Geometry check sheet. Reference: the model listing, model coordinates, mm. A direction names the side the tool comes from. Coordinates: 2 decimals unless noted, no trailing zeros. Loops run counter-clockwise (first coordinate to the right, second up) from the corner with the lowest first, then second, coordinate; pieces in that order, holes last. Notation, with made-up numbers: (-22.75, 19) - (21.25, 19) arc R20 cw to (21.25, 56) - close; hole circle Ø7 at (-4.75, 72). An arc over 180 degrees is marked (long way). Write each question's results on one line, items separated by ' | '. Start each with the question number.
(1) Mould release check, pull along Y, two halves, no side actions. Record for faces 3 (the face through (31, 9.76, 11.83)), 4 (the face through (-25, 0, 23)), 5 (the face through (-29, -9, -3)): pulls with the +Y half, pulls with the -Y half, needs draft (parallel to the pull), parting line crosses it, or undercut.
(2) Sectioned sample at C-C (z = 8.75). Enter the section's corners in (x, y), plus the area to 3 significant figures.
(3) Access from +Z, -Z, +X, -X, +Y, -Y to the whole of each face (thin tool, end or side, straight path). Record for faces 1 (the face through (-28, 0, 21.5)), 2 (the face through (25, 0, 23)).
(4) Sectioned sample at D-D (y = 23). Enter the section's corners in (x, z).
(5) Material ranges on probe 1 along Y at (x, z) = (0, 11.5); probe 2 along Y at (x, z) = (27.5, 14.5); probe 3 along Z at (x, y) = (23.5, 24.5), recorded low to high.
(6) Go/stop test with flat-tipped pins: pin 1 Ø2.5 at (x, y) = (28.5, -1) entering from -Z; pin 2 Ø2 at (x, z) = (26.5, 22.5) entering from +Y; pin 3 Ø0.8 at (x, z) = (0, 23) entering from +Y. Record where each tip stops, or that it passes through.
(7) Sectioned sample at A-A (y = 0). Enter the section's corners in (x, z).
from build123d import *

# Parameters (mm, degrees)
F0_R     = 42.5
F0_R_2   = 32.5
F0_R_3   = 30
F1_DEPTH = 3
F2_DEPTH = 24
F4_DEPTH = 2.5


with BuildPart() as f1:
    # F0 (on Top) → F1 (new body)
    with BuildSketch(Plane.XY):
        Circle(F0_R)
        Circle(F0_R_2, mode=Mode.SUBTRACT)
        Circle(F0_R_2)
        Circle(F0_R_3, mode=Mode.SUBTRACT)
    extrude(amount=-F1_DEPTH)

    # F0 (on Top) → F2 (join)
    with BuildSketch(Plane.XY):
        Circle(F0_R_2)
        Circle(F0_R_3, mode=Mode.SUBTRACT)
    extrude(amount=F2_DEPTH)

    # F3 (on face) → F4 (join)
    with BuildSketch(Plane.XY.offset(24)):
        with BuildLine():
            Line((25, -2.5), (29.8956518578, -2.5))
            ThreePointArc((29.8956518578, -2.5), (29.9739016123, -1.2510883797), (30, 0))
            ThreePointArc((30, 0), (29.9739016123, 1.2510883797), (29.8956518578, 2.5))
            Line((29.8956518578, 2.5), (25, 2.5))
            Line((25, 2.5), (25, -2.5))
        make_face()
        with BuildLine():
            ThreePointArc((-30, 0), (-29.9739016123, -1.2510883797), (-29.8956518578, -2.5))
            Line((-29.8956518578, -2.5), (-25, -2.5))
            Line((-25, -2.5), (-25, 2.5))
            Line((-25, 2.5), (-29.8956518578, 2.5))
            ThreePointArc((-29.8956518578, 2.5), (-29.9739016123, 1.2510883797), (-30, 0))
        make_face()
        with BuildLine():
            Line((2.5, 25), (2.5, 29.8956518578))
            ThreePointArc((2.5, 29.8956518578), (1.2510883797, 29.9739016123), (0, 30))
            ThreePointArc((0, 30), (-1.2510883797, 29.9739016123), (-2.5, 29.8956518578))
            Line((-2.5, 29.8956518578), (-2.5, 25))
            Line((-2.5, 25), (2.5, 25))
        make_face()
        with BuildLine():
            ThreePointArc((0, -30), (1.2510883797, -29.9739016123), (2.5, -29.8956518578))
            Line((2.5, -29.8956518578), (2.5, -25))
            Line((2.5, -25), (-2.5, -25))
            Line((-2.5, -25), (-2.5, -29.8956518578))
            ThreePointArc((-2.5, -29.8956518578), (-1.2510883797, -29.9739016123), (0, -30))
        make_face()
    extrude(amount=-F4_DEPTH)


solid = f1.part
Outcome:
1) face 3: parting line crosses it | face 4: undercut | face 5: needs draft
2) outline: circle Ø65 at (0, 0); hole circle Ø60 at (0, 0) | area: 491 mm2
3) face 1: -Z | face 2: +Z, -Z
4) outline: (-35.74, -3) - (-19.26, -3) - (-19.26, 24) - (-22.96, 24) - (-22.96, 0) - (-35.74, 0) - close; (19.26, -3) - (35.74, -3) - (35.74, 0) - (22.96, 0) - (22.96, 24) - (19.26, 24) - close
5) probe 1: y = -32.5 to -30, 30 to 32.5 | probe 2: y = -17.32 to -11.99, 11.99 to 17.32 | probe 3: z = -3 to 0
6) pin 1: stops at z = 21.5 | pin 2: stops at y = 20.15 | pin 3: stops at y = 32.5
7) outline: (-42.5, -3) - (-30, -3) - (-30, 21.5) - (-25, 21.5) - (-25, 24) - (-32.5, 24) - (-32.5, 0) - (-42.5, 0) - close; (25, 21.5) - (30, 21.5) - (30, -3) - (42.5, -3) - (42.5, 0) - (32.5, 0) - (32.5, 24) - (25, 24) - close
